Model file for the job. Use its own axes, mm. Give positions to 0.01 mm unless a question says otherwise; leave off trailing zeros. Order: outer loops, then holes, each group sorted by start corner. A loop starts at its lowest first (then second) coordinate and runs counter-clockwise, first axis right, second up. Notation, with made-up numbers: (21, 26) -> (53, 26) arc R17 ccw to (53, 31) -> close; hole circle Ø11 at (55.5, 69). An arc over 180 degrees is marked (long way). Use CSV: the item, a comma, the result in double quotes. Start each with the question number.
1. Wall check: line 1 (X direction, y = 19.3, z = -231); line 2 (X direction, y = 16.2, z = -228); line 3 (Z direction, x = -146.5, y = 17.8). Give the ranges that are in metal, low to high. Write a range as from..to.
2. Drop flat-ended pins along their axis: pin 1 (7 mm diameter, centred on x = -81.64, z = -228.79, fed in from -Y); pin 2 (1.5 mm diameter, centred on y = 19, z = -235.5, fed in from +X); pin 3 (1.5 mm diameter, centred on x = -103.5, y = 18.5, fed in from -Z). Give the stop position or say it passes through.
3. Cut at C-C on y = 18.5. List the corners of the cut face in (x, z), then the cut area to 3 significant figures.
4. Cut at B-B on x = -83. List the corners of the cut face in (y, z).
5. Cut at D-D on x = -95. List the corners of the cut face in (y, z), then the cut area to 3 significant figures.
6. Cut at A-A on z = -247. List the corners of the cut face in (x, y), then the cut area to 3 significant figures.
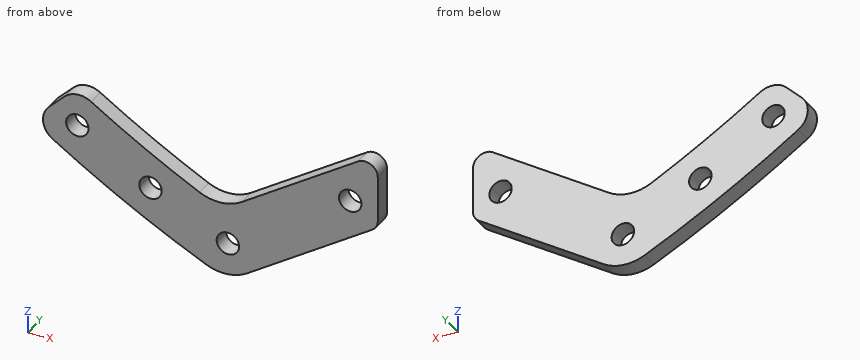
```python
from build123d import *

# Parameters (mm, degrees)
SKETCH_1_R               = 275
SKETCH_1_R_2             = 255
EXTRUDE_1_DEPTH          = 10
EXTRUDE_2_DEPTH          = 10
SKETCH_8_R               = 2.65
CUT_EXTRUDE_1_DEPTH      = 21
SKETCH_9_OUTSIDE_W       = 707.614
SKETCH_9_OUTSIDE_H       = 707.614
CUT_EXTRUDE_2_DEPTH      = 21
SKETCH_10_W              = 90.654248201
SKETCH_10_H              = 12
CUT_EXTRUDE_3_DEPTH      = 519.420037555
CUT_EXTRUDE_3_DEPTH_BACK = 245.939436413
FILLET_1_R               = 3
FILLET_2_R               = 10
FILLET_3_R               = 5
SKETCH_11_W              = 550
SKETCH_11_H              = 20
CUT_EXTRUDE_4_DEPTH      = 519.420037555
CUT_EXTRUDE_4_DEPTH_BACK = 245.939436413
CUT_EXTRUDE_5_DEPTH      = 11
FILLET_4_R               = 3


with BuildPart() as part:
    # 草图1 → 凸台-拉伸1 (new body)
    with BuildSketch(Plane(origin=(0, 0, 0), x_dir=(1, 0, 0), z_dir=(0, 1, 0))):
        Circle(SKETCH_1_R)
        Circle(SKETCH_1_R_2, mode=Mode.SUBTRACT)
    extrude(amount=EXTRUDE_1_DEPTH)

    # 草图11 → 切除-拉伸4 (cut, two sides)
    with BuildSketch(Plane(origin=(76.33674701, 0, -113.448714652), x_dir=(0.829665535, 0, 0.558260781), z_dir=(-0.558260781, 0, 0.829665535))) as cut_extrude_4_sk:
        Rectangle(SKETCH_11_W, SKETCH_11_H)
    extrude(amount=CUT_EXTRUDE_4_DEPTH, mode=Mode.SUBTRACT)
    extrude(cut_extrude_4_sk.sketch, amount=-CUT_EXTRUDE_4_DEPTH_BACK, mode=Mode.SUBTRACT)


with BuildPart() as body_2:
    # 草图2 → 凸台-拉伸2 (new body)
    with BuildSketch(Plane(origin=(0, 10, 0), x_dir=(1, 0, 0), z_dir=(0, 1, 0))):
        with BuildLine():
            Line((-110.525139894, 257.262887824), (-25.423255477, 200))
            Line((-25.423255477, 200), (0, 200))
            Line((0, 200), (25.423255477, 200))
            Line((25.423255477, 200), (110.525139894, 257.262887824))
            ThreePointArc((110.525139894, 257.262887824), (197.989898732, 197.989898732), (257.262887824, 110.525139894))
            Line((257.262887824, 110.525139894), (200, 25.423255477))
            Line((200, 25.423255477), (200, 0))
            Line((200, 0), (200, -25.423255477))
            Line((200, -25.423255477), (257.262887824, -110.525139894))
            ThreePointArc((257.262887824, -110.525139894), (197.989898732, -197.989898732), (110.525139894, -257.262887824))
            Line((110.525139894, -257.262887824), (25.423255477, -200))
            Line((25.423255477, -200), (0, -200))
            Line((0, -200), (-25.423255477, -200))
            Line((-25.423255477, -200), (-110.525139894, -257.262887824))
            ThreePointArc((-110.525139894, -257.262887824), (-197.989898732, -197.989898732), (-257.262887824, -110.525139894))
            Line((-257.262887824, -110.525139894), (-200, -25.423255477))
            Line((-200, -25.423255477), (-200, 25.423255477))
            Line((-200, 25.423255477), (-257.262887824, 110.525139894))
            ThreePointArc((-257.262887824, 110.525139894), (-197.989898732, 197.989898732), (-110.525139894, 257.262887824))
        make_face()
        with BuildLine():
            Line((0, 185), (30, 185))
            Line((30, 185), (111.993839361, 240.171563565))
            ThreePointArc((111.993839361, 240.171563565), (187.383297014, 187.383297014), (240.171563565, 111.993839361))
            Line((240.171563565, 111.993839361), (185, 30))
            Line((185, 30), (185, 0))
            Line((185, 0), (185, -30))
            Line((185, -30), (240.171563565, -111.993839361))
            ThreePointArc((240.171563565, -111.993839361), (187.383297014, -187.383297014), (111.993839361, -240.171563565))
            Line((111.993839361, -240.171563565), (30, -185))
            Line((30, -185), (0, -185))
            Line((0, -185), (-30, -185))
            Line((-30, -185), (-111.993839361, -240.171563565))
            ThreePointArc((-111.993839361, -240.171563565), (-187.383297014, -187.383297014), (-240.171563565, -111.993839361))
            Line((-240.171563565, -111.993839361), (-185, -30))
            Line((-185, -30), (-185, 30))
            Line((-185, 30), (-240.171563565, 111.993839361))
            ThreePointArc((-240.171563565, 111.993839361), (-187.383297014, 187.383297014), (-111.993839361, 240.171563565))
            Line((-111.993839361, 240.171563565), (-30, 185))
            Line((-30, 185), (0, 185))
        make_face(mode=Mode.SUBTRACT)
    extrude(amount=EXTRUDE_2_DEPTH)

    # 草图8 → 切除-拉伸1 (cut, through all)
    with BuildSketch(Plane(origin=(0, 20, 0), x_dir=(1, 0, 0), z_dir=(0, 1, 0))):
        with Locations((-10, 192.5)):
            Circle(SKETCH_8_R)
        with Locations((10, 192.5)):
            Circle(SKETCH_8_R)
        with Locations((-10, -192.5)):
            Circle(SKETCH_8_R)
        with Locations((10, -192.5)):
            Circle(SKETCH_8_R)
        with Locations((192.5, 10)):
            Circle(SKETCH_8_R)
        with Locations((192.5, -10)):
            Circle(SKETCH_8_R)
        with Locations((-192.5, 10)):
            Circle(SKETCH_8_R)
        with Locations((-192.5, -10)):
            Circle(SKETCH_8_R)
        with Locations((-110.525139894, 248.223100485)):
            Circle(SKETCH_8_R)
        with Locations((-27.711627738, 192.5)):
            Circle(SKETCH_8_R)
        with Locations((-44.304938442, 203.665215623)):
            Circle(SKETCH_8_R)
        with Locations((-56.749921469, 212.03912734)):
            Circle(SKETCH_8_R)
        with Locations((-69.194904497, 220.413039057)):
            Circle(SKETCH_8_R)
        with Locations((-81.639887524, 228.786950774)):
            Circle(SKETCH_8_R)
        with Locations((-146.077022117, 230.028561882)):
            Circle(SKETCH_8_R)
        with Locations((-164.415519771, 217.299729706)):
            Circle(SKETCH_8_R)
        with Locations((-183.638937552, 201.316607082)):
            Circle(SKETCH_8_R)
        with Locations((-201.316607082, 183.638937552)):
            Circle(SKETCH_8_R)
        with Locations((-217.299729706, 164.415519771)):
            Circle(SKETCH_8_R)
        with Locations((-230.028561882, 146.077022117)):
            Circle(SKETCH_8_R)
        with Locations((-128.811575358, 240.123330241)):
            Circle(SKETCH_8_R)
        with Locations((-240.123330241, 128.811575358)):
            Circle(SKETCH_8_R)
        with Locations((-228.786950774, 81.639887524)):
            Circle(SKETCH_8_R)
        with Locations((-220.413039057, 69.194904497)):
            Circle(SKETCH_8_R)
        with Locations((-212.03912734, 56.749921469)):
            Circle(SKETCH_8_R)
        with Locations((-203.665215623, 44.304938442)):
            Circle(SKETCH_8_R)
        with Locations((-192.5, 27.711627738)):
            Circle(SKETCH_8_R)
        with Locations((-248.223100485, 110.525139894)):
            Circle(SKETCH_8_R)
        with Locations((192.5, 27.711627738)):
            Circle(SKETCH_8_R)
        with Locations((248.223100485, 110.525139894)):
            Circle(SKETCH_8_R)
        with Locations((203.665215623, 44.304938442)):
            Circle(SKETCH_8_R)
        with Locations((212.03912734, 56.749921469)):
            Circle(SKETCH_8_R)
        with Locations((220.413039057, 69.194904497)):
            Circle(SKETCH_8_R)
        with Locations((228.786950774, 81.639887524)):
            Circle(SKETCH_8_R)
        with Locations((240.123330241, 128.811575358)):
            Circle(SKETCH_8_R)
        with Locations((230.028561882, 146.077022117)):
            Circle(SKETCH_8_R)
        with Locations((128.811575358, 240.123330241)):
            Circle(SKETCH_8_R)
        with Locations((201.316607082, 183.638937552)):
            Circle(SKETCH_8_R)
        with Locations((183.638937552, 201.316607082)):
            Circle(SKETCH_8_R)
        with Locations((164.415519771, 217.299729706)):
            Circle(SKETCH_8_R)
        with Locations((146.077022117, 230.028561882)):
            Circle(SKETCH_8_R)
        with Locations((81.639887524, 228.786950774)):
            Circle(SKETCH_8_R)
        with Locations((69.194904497, 220.413039057)):
            Circle(SKETCH_8_R)
        with Locations((56.749921469, 212.03912734)):
            Circle(SKETCH_8_R)
        with Locations((44.304938442, 203.665215623)):
            Circle(SKETCH_8_R)
        with Locations((110.525139894, 248.223100485)):
            Circle(SKETCH_8_R)
        with Locations((27.711627738, 192.5)):
            Circle(SKETCH_8_R)
        with Locations((217.299729706, 164.415519771)):
            Circle(SKETCH_8_R)
    extrude(amount=-CUT_EXTRUDE_1_DEPTH, mode=Mode.SUBTRACT)

    # 草图9 outside → 切除-拉伸2 (cut, through all)
    with BuildSketch(Plane(origin=(0, 20, 0), x_dir=(1, 0, 0), z_dir=(0, 1, 0))):
        Rectangle(SKETCH_9_OUTSIDE_W, SKETCH_9_OUTSIDE_H)
        with BuildLine():
            Line((-157.049761777, 231.808913387), (-146.237600169, 220.996751779))
            ThreePointArc((-146.237600169, 220.996751779), (-129.47118383, 231.218971016), (-111.993839361, 240.171563565))
            Line((-111.993839361, 240.171563565), (-64.194904497, 208.008879225))
            Line((-64.194904497, 208.008879225), (-64.194904497, 226.088453902))
            Line((-64.194904497, 226.088453902), (-110.525139894, 257.262887824))
            ThreePointArc((-110.525139894, 257.262887824), (-134.391436501, 245.639861983), (-157.049761777, 231.808913387))
        make_face(mode=Mode.SUBTRACT)
    extrude(amount=-CUT_EXTRUDE_2_DEPTH, mode=Mode.SUBTRACT)

    # 草图10 → 切除-拉伸3 (cut, two sides)
    with BuildSketch(Plane(origin=(76.33674701, 0, -113.448714652), x_dir=(0.829665535, 0, 0.558260781), z_dir=(-0.558260781, 0, 0.829665535))) as cut_extrude_3_sk:
        with Locations((-226.995793353, 10)):
            Rectangle(SKETCH_10_W, SKETCH_10_H)
    extrude(amount=CUT_EXTRUDE_3_DEPTH, mode=Mode.SUBTRACT)
    extrude(cut_extrude_3_sk.sketch, amount=-CUT_EXTRUDE_3_DEPTH_BACK, mode=Mode.SUBTRACT)

    # 圆角1
    fillet_1_edges = [body_2.edges().sort_by_distance(p)[0] for p in [
        (-64.194904497, 15, -208.008879225),
    ]]
    fillet(fillet_1_edges, radius=FILLET_1_R)

    # 圆角2
    fillet_2_edges = [body_2.edges().sort_by_distance(p)[0] for p in [
        (-110.525139894, 18, -257.262887824),
        (-111.993839361, 18, -240.171563565),
    ]]
    fillet(fillet_2_edges, radius=FILLET_2_R)

    # 圆角3
    fillet_3_edges = [body_2.edges().sort_by_distance(p)[0] for p in [
        (-157.049761777, 18, -231.808913387),
        (-146.237600169, 18, -220.996751779),
        (-64.194904497, 15, -226.088453902),
    ]]
    fillet(fillet_3_edges, radius=FILLET_3_R)

    # 草图12 → 切除-拉伸5 (cut, through all)
    with BuildSketch(Plane(origin=(0, 20, 0), x_dir=(1, 0, 0), z_dir=(0, 1, 0))):
        Polygon((-75.139887524, 233.453053871), (-75.139887524, 215.373479194), (-74.80041279, 205.67344135), (-60.747401583, 205.67344135), (-60.747401583, 233.453053871), align=None)
    extrude(amount=-CUT_EXTRUDE_5_DEPTH, mode=Mode.SUBTRACT)

    # 圆角4
    fillet_4_edges = [body_2.edges().sort_by_distance(p)[0] for p in [
        (-75.139887524, 18, -215.373479194),
        (-75.139887524, 18, -233.453053871),
    ]]
    fillet(fillet_4_edges, radius=FILLET_4_R)


solid = body_2.part
```
Verdict:
1,line 1,"-154.19..-148.54, -143.61..-129.86, -98.36..-83.1, -80.18..-75.14"
1,line 2,"-153.17..-147.78, -144.37..-135.06, -93.9..-84.17, -79.11..-75.14"
1,line 3,"-238.62..-232.64, -227.41..-222.49"
2,pin 1,"y = 16"
2,pin 2,"x = -77.07"
2,pin 3,"z = -253.04"
3,outline,"(-152.72, -227.48) arc R5 ccw to (-151.9, -235.22) arc R280 ccw to (-115.66, -254.99) arc R10 ccw to (-105.95, -254.18) -> (-76.47, -234.34) arc R3 ccw to (-75.14, -231.86) -> (-75.14, -221.01) arc R3 ccw to (-79.81, -218.52) -> (-107.25, -236.98) arc R10 cw to (-117.25, -237.65) arc R265 cw to (-142.87, -223.19) arc R5 ccw to (-149.1, -223.86) -> close; hole circle Ø5.3 at (-146.08, -230.03); hole circle Ø5.3 at (-128.81, -240.12); hole circle Ø5.3 at (-110.53, -248.22); hole circle Ø5.3 at (-81.64, -228.79)"
3,area,"1,240 mm^2"
4,outline,"(16, -238.74) -> (20, -238.74) -> (20, -231.06) -> (16, -231.06) -> close; (16, -226.51) -> (20, -226.51) -> (20, -220.66) -> (16, -220.66) -> close"
5,outline,"(16, -246.82) -> (20, -246.82) -> (20, -228.74) -> (16, -228.74) -> close"
5,area,"72.3 mm^2"
6,outline,"(-131.87, 16) -> (-112.88, 16) -> (-112.88, 20) -> (-131.87, 20) -> close; (-108.17, 16) -> (-95.27, 16) -> (-95.27, 20) -> (-108.17, 20) -> close"
6,area,"128 mm^2"
